The drawing under review shows one solid part. Ordinate dimensions are in mm from its lowest x, y, z. Give positions to 0.01 mm unless a question says otherwise; leave off trailing zeros. Write each loop counter-clockwise with the first axis right and the second up, starting at its lowest first coordinate (ties: lowest second). Pieces come first, ordered by that corner, then holes. Notation, with made-up numbers: (-24, -20) -> (30, -20) arc R21 ccw to (30, 4) -> close; hole circle Ø5 at (-22, -36.5). An arc over 180 degrees is marked (long way). Use CSV: the item, a comma, the result in double quotes.
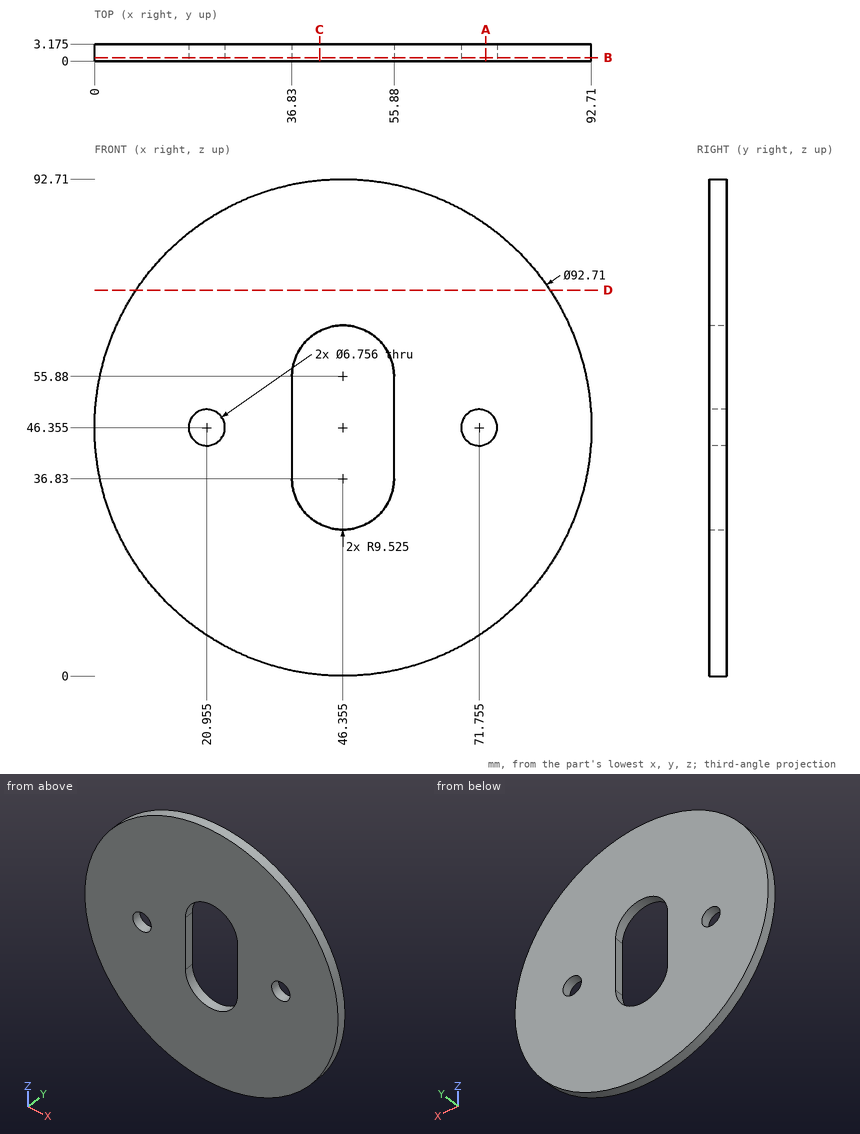
(1) Take a section at C-C (x = 42). Write out the cut boundary in (y, z) (1 decimal).
Established:
outline,"(0, 0.2) -> (3.2, 0.2) -> (3.2, 28.4) -> (0, 28.4) -> close; (0, 64.4) -> (3.2, 64.4) -> (3.2, 92.5) -> (0, 92.5) -> close"
(2) Take a section at B-B (y = 0.65). State how many separate pieces and enclosed holes the cut face has, then the cut area to 3 significant figures.
Established:
separate pieces,"1"
enclosed holes,"3"
area,"6,030 mm2"
(3) Take a section at D-D (z = 72). Write out the cut boundary in (x, y) (1 decimal), then the cut area to 3 significant figures.
Established:
outline,"(7.7, 0) -> (85, 0) -> (85, 3.2) -> (7.7, 3.2) -> close"
area,"245 mm2"
(4) For line 1 along X through (y, z) = (3, 48) (1 decimal); line 2 along Z through (x, y) = (46, 0.85); line 3 along Z through (x, y) = (47.5, 2.5) (1 decimal), list the stretches that pass through material, from the lowest coordinate up. Write a range as [from, to].
Established:
line 1,"x = [0, 18], [23.9, 36.8], [55.9, 68.8], [74.7, 92.7]"
line 2,"z = [0, 27.31], [65.4, 92.71]"
line 3,"z = [0, 27.4], [65.3, 92.7]"
(5) Take a section at A-A (x = 73). Write out the cut boundary in (y, z) (1 decimal), then the cut area to 3 significant figures.
Established:
outline,"(0, 8.4) -> (3.2, 8.4) -> (3.2, 43.2) -> (0, 43.2) -> close; (0, 49.5) -> (3.2, 49.5) -> (3.2, 84.3) -> (0, 84.3) -> close"
area,"221 mm2"
(6) Clearance check with flat-ended pins moving along their axes: pin 1 (1.6 mm diameter, centred on y = 2.5, z = 46, fed in from +X); pin 2 (1 mm diameter, centred on y = 1.5, z = 81, fed in from +X) (1 decimal); pin 3 (4 mm diameter, centred on x = 20.955, z = 46.355, fed in from -Y); pin 4 (1 mm diameter, centred on x = 33.5, y = 0.5, fed in from -Z). State where each tip first meets the part, or that it passes through.
Established:
pin 1,"stops at x = 92.71"
pin 2,"stops at x = 77.7"
pin 3,"passes through"
pin 4,"stops at z = 1.68"
